Model file for the job. Use its own axes, mm. A direction names the side the tool comes from. Coordinates: 2 decimals unless noted, no trailing zeros. Loops run counter-clockwise (first coordinate to the right, second up) from the corner with the lowest first, then second, coordinate; pieces in that order, holes last.
from build123d import *

# Parameters (mm, degrees)
CROQUIS1_W              = 215
CROQUIS1_H              = 160
CROQUIS1_R              = 1
SALIENTE_EXTRUIR1_DEPTH = 8
CROQUIS1_3_W            = 215
CROQUIS1_3_H            = 23
CROQUIS1_3_R            = 1
SALIENTE_EXTRUIR2_DEPTH = 25


with BuildPart() as part:
    # Croquis1 → Saliente-Extruir1 (new body)
    with BuildSketch(Plane.XY):
        with Locations((73.249006664, -76.149492386)):
            Rectangle(CROQUIS1_W, CROQUIS1_H)
        with Locations((5.749006664, -146.149492386)):
            Circle(CROQUIS1_R, mode=Mode.SUBTRACT)
        with Locations((170.749006664, -146.149492386)):
            Circle(CROQUIS1_R, mode=Mode.SUBTRACT)
    extrude(amount=SALIENTE_EXTRUIR1_DEPTH)

    # Croquis1_3 → Saliente-Extruir2 (add)
    with BuildSketch(Plane.XY):
        with Locations((73.249006664, 15.350507614)):
            Rectangle(CROQUIS1_3_W, CROQUIS1_3_H)
        with Locations((5.749006664, 16.850507614)):
            Circle(CROQUIS1_3_R, mode=Mode.SUBTRACT)
        with Locations((170.749006664, 16.850507614)):
            Circle(CROQUIS1_3_R, mode=Mode.SUBTRACT)
    extrude(amount=SALIENTE_EXTRUIR2_DEPTH)


solid = part.part
Q1. Slice it at B-B (z = 12). List the corners of the cut face in (x, y), and give its area (3 significant figures).
Answers:
outline: (-34.25, 3.85) - (180.75, 3.85) - (180.75, 26.85) - (-34.25, 26.85) - close; hole circle Ø2 at (5.75, 16.85); hole circle Ø2 at (170.75, 16.85)
area: 4,940 mm2
Q2. Which spindle directions (+Z, -Z, +X, -X, +Y, -Y) get a long thin tool onto all of the face, cutting with end or side? Do faces 1 (the flat face through (72, -156.149, 4)), 2 (the flat face through (72, 3.851, 16)). Say none if no direction does.
Answers:
face 1: +Z, -Z, +X, -X, -Y
face 2: +Z, +X, -X, -Y
Q3. Flat gauge pins, fed straight in: P1, Ø2.5, axis at x = 170.75, y = -146.15, coming from the +Z side; P2, Ø8.5, axis at x = 49, z = 19.5, coming from the -Y side. Where does each tip first touch, or does it go through?
Answers:
P1: stops at z = 8
P2: stops at y = 3.85
Q4. Drill centre lines: line 1 (Z direction, x = -23, y = -61); line 2 (Y direction, x = 41.5, z = 20.5). Where is each one in solid material? Low to high.
Answers:
line 1: z = 0 to 8
line 2: y = 3.85 to 26.85
Q5. Slice it at A-A (x = 20). List the corners of the cut face in (y, z), and give its area (4 significant figures).
Answers:
outline: (-156.15, 0) - (26.85, 0) - (26.85, 25) - (3.85, 25) - (3.85, 8) - (-156.15, 8) - close
area: 1,855 mm2
Q6. Slice it at C-C (y = -114.5). List the corners of the cut face in (x, z), and give its area (3 significant figures).
Answers:
outline: (-34.25, 0) - (180.75, 0) - (180.75, 8) - (-34.25, 8) - close
area: 1,720 mm2
